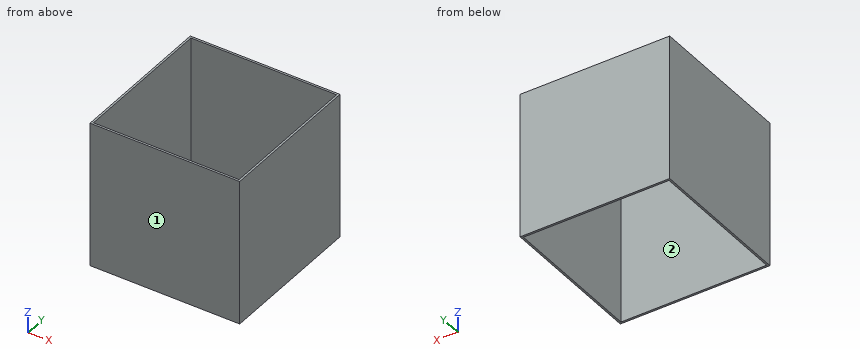
Autodesk Inventor part; units mm, degrees
ref_plane "YZ Plane" through (0, 0, 0) normal (1, 0, 0) x (0, 1, 0)
ref_plane "XZ Plane" through (0, 0, 0) normal (0, 1, 0) x (-1, 0, 0)
ref_plane "XY Plane" through (0, 0, 0) normal (0, 0, 1) x (1, 0, 0)
sketch "Sketch1" plane through (0, 0, 0) normal (0, 0, 1) x (1, 0, 0)
  line L0 (0, 0) -> (469.9, 0)
  line L1 (469.9, 0) -> (469.9, 469.9)
  line L2 (469.9, 469.9) -> (0, 469.9)
  line L3 (0, 469.9) -> (0, 0)
  dimension "d0" = 469.9
  dimension "d1" = 469.9
extrude "Extrusion1" add sketch "Sketch1" along normal blind 457.2
shell "Shell1" thickness 6.35 removed faces 2 at (156.6333, 313.2667, 0) at (156.6333, 313.2667, 457.2)
equation "\"d2\" = size"
equation "\"size\" = 457.2"
properties part number "Sizing Tool-01"
Geometry: final body of the model. Coordinates: model frame, mm. Face numbers are marked on the shaded views. A direction names the side the tool comes from. Round coordinates to 2 decimals unless told otherwise and drop trailing zeros. Write each loop counter-clockwise with the first axis right and the second up, starting at its lowest first coordinate (ties: lowest second). Pieces come first, ordered by that corner, then holes. Notation, with made-up numbers: M 77.25,-1 L 130.25,-1 A16 ccw 130.25,12 Z; hole C -10,53 d2. An arc over 180 degrees is marked long. Answer in a Markdown table with one row per item. Add a question column.
(1) Cut plane B-B, the plane z = 208. Return the cut outline in (x, y), then the cut area to 3 significant figures.
(2) Reachability of the marked faces 1 and 2 from +Z, -Z, +X, -X, +Y, -Y: full face, straight path, thin tool, end or side. Return the list, or none.
(3) Cut plane A-A, the plane x = 349.5. Return the cut outline in (y, z), then the cut area to 3 significant figures.
(4) Ray query, L1, parallel to Y at x = 182.5, z = 158.5. Return the intervals inside material, ascending.
Established:
| question | item | result |
|---|---|---|
| 1 | outline | M 0,0 L 469.9,0 L 469.9,469.9 L 0,469.9 Z; hole M 6.35,6.35 L 463.55,6.35 L 463.55,463.55 L 6.35,463.55 Z |
| 1 | area | 11,800 mm² |
| 2 | face 1 | +Z, -Z, +X, -X, -Y |
| 2 | face 2 | +Z, -Z |
| 3 | outline | M 0,0 L 6.35,0 L 6.35,457.2 L 0,457.2 Z; M 463.55,0 L 469.9,0 L 469.9,457.2 L 463.55,457.2 Z |
| 3 | area | 5,810 mm² |
| 4 | L1 | 0 to 6.35, 463.55 to 469.9 |
